Geometry: final body of the model. Coordinates: model frame, mm. Give positions to 0.01 mm unless a question says otherwise; leave off trailing zeros. Write each loop counter-clockwise with the first axis right and the second up, starting at its lowest first coordinate (ties: lowest second). Pieces come first, ordered by that corner, then holes. Notation, with made-up numbers: (50, 42) -> (83, 42) arc R23 ccw to (83, 65) -> close; hole circle Ø5 at (0, 7). An arc over 180 degrees is marked (long way). Use CSV: the item, a comma, the result in double quotes. Start each with the question number.
1) Section D-D (x = 1). Output: boundary loops of the cut face in (y, z) (3 decimals), plus the area to 3 significant figures.
2) Section B-B (x = 6.35). Output: boundary loops of the cut face in (y, z) (1 decimal).
3) Material intervals for line 1 (Y direction, x = 6.35, z = 1.15); line 2 (Y direction, x = 7.75, z = 0.45); line 3 (X direction, y = 6.5, z = 3.05), sorted ascending. Write a range as [from, to].
4) Section C-C (y = 6.35). Output: boundary loops of the cut face in (x, z) (1 decimal), plus the area to 3 significant figures.
5) Contact query for a flat-ended pin moving along its axis: P1, Ø2.5, axis at x = 6.35, y = 6.35, coming from the -Z side. Output: stop coordinate, or through.
6) Section A-A (z = 2.25). Count the separate pieces of the cut face and the enclosed holes in it, plus the area to 3 significant figures.
7) Draft query along Y for faces 1 (the face through (6, 0, 2)), 2 (the face through (12.7, 25, 2)), 3 (the face through (6, 42.9, 1.6)). Return one class per face: pulls with the +Y half, pulls with the -Y half, needs draft (parallel to the pull), parting line crosses it, or undercut.
```python
from build123d import *

# Parameters (mm, degrees)
F0_W     = 12.7
F0_H     = 50.8
F0_R     = 1.5875
F1_DEPTH = 3.175
F2_R     = 5.08


# Not quite as in the source:
# - a length typed as a fraction of an inch, garbled in the dataset ("3 / 203.2 mm" for 3/8 in), is restored


with BuildPart() as f1:
    # F0 (on Top) → F1 (new body)
    with BuildSketch(Plane.XY):
        with Locations((6.35, 25.4)):
            Rectangle(F0_W, F0_H)
        with Locations((6.35, 6.35)):
            Circle(F0_R, mode=Mode.SUBTRACT)
        with Locations((6.35, 44.45)):
            Circle(F0_R, mode=Mode.SUBTRACT)
    extrude(amount=F1_DEPTH)

    # F2
    f2_edges = [f1.edges().sort_by_distance(p)[0] for p in [
        (12.7, 0, 1.5875),
        (0, 0, 1.5875),
        (12.7, 50.8, 1.5875),
        (0, 50.8, 1.5875),
    ]]
    fillet(f2_edges, radius=F2_R)


solid = f1.part
```
Answers follow:
1,outline,"(2.053, 0) -> (48.747, 0) -> (48.747, 3.175) -> (2.053, 3.175) -> close"
1,area,"148 mm^2"
2,outline,"(0, 0) -> (4.8, 0) -> (4.8, 3.2) -> (0, 3.2) -> close; (7.9, 0) -> (42.9, 0) -> (42.9, 3.2) -> (7.9, 3.2) -> close; (46, 0) -> (50.8, 0) -> (50.8, 3.2) -> (46, 3.2) -> close"
3,line 1,"y = [0, 4.76], [7.94, 42.86], [46.04, 50.8]"
3,line 2,"y = [0, 5.6], [7.1, 43.7], [45.2, 50.8]"
3,line 3,"x = [0, 4.77], [7.93, 12.7]"
4,outline,"(0, 0) -> (4.8, 0) -> (4.8, 3.2) -> (0, 3.2) -> close; (7.9, 0) -> (12.7, 0) -> (12.7, 3.2) -> (7.9, 3.2) -> close"
4,area,"30.2 mm^2"
5,P1,"passes through"
6,separate pieces,"1"
6,enclosed holes,"2"
6,area,"607 mm^2"
7,face 1,"pulls with the -Y half"
7,face 2,"needs draft"
7,face 3,"undercut"
